For this review, take the finished solid that the model builds, in its own axes (mm). Coordinates: 2 decimals unless noted, no trailing zeros. Loops run counter-clockwise (first coordinate to the right, second up) from the corner with the lowest first, then second, coordinate; pieces in that order, holes last. Notation, with made-up numbers: (67, 9.5) -> (83, 9.5) arc R12 ccw to (83, 26.5) -> close; hole circle Ø8 at (-2, 28.25). An arc over 180 degrees is marked (long way). Use a Markdown table: item, result.
from build123d import *

# Parameters (mm, degrees)
SKETCH1_2_R                 = 1.6383
BOSS_EXTRUDE2_DEPTH         = 1.575
SKETCH2_W                   = 14.080651801
SKETCH2_H                   = 7.11628052
SKETCH2_W_2                 = 15.007196354
SKETCH2_H_2                 = 9.421332762
CUT_EXTRUDE1_DEPTH          = 65.400942629
ADDITIONAL_PCB_MATERIAL_W   = 2.649520344
ADDITIONAL_PCB_MATERIAL_H   = 65.213315835
ADDITIONAL_PCB_MATERIAL_W_2 = 1.5
ADDITIONAL_PCB_MATERIAL_H_2 = 65.299191064
BOSS_EXTRUDE3_DEPTH         = 1.575
SKETCH3_W                   = 46.818
SKETCH3_H                   = 1
BOSS_EXTRUDE4_DEPTH         = 1.575
SKETCH4_W                   = 2
SKETCH4_H                   = 2.5
CUT_EXTRUDE2_DEPTH          = 65.400942629
SKETCH5_W                   = 2.5
SKETCH5_H                   = 18.09999695
SKETCH5_H_2                 = 19.499999394
BOSS_EXTRUDE5_DEPTH         = 1.575
SKETCH7_W                   = 9.5
SKETCH7_H                   = 1.20600305
CUT_EXTRUDE3_DEPTH          = 65.400942629
SKETCH26_W                  = 2.575
SKETCH26_H                  = 5
CUT_EXTRUDE4_DEPTH          = 10


with BuildPart() as part:
    # Sketch1_2 → Boss-Extrude2 (new body)
    with BuildSketch(Plane(origin=(0, 0, 0), x_dir=(1, 0, 0), z_dir=(0, 1, 0))):
        with BuildLine():
            Line((-38.39500299, 29.999999735), (-42.73000299, 29.999999735))
            Line((-42.73000299, 29.999999735), (-43.011025994, 30.003097626))
            ThreePointArc((-43.011025994, 30.003097626), (-43.710996344, 30.299838092), (-44.000003042, 31.003036872))
            Line((-44.000003042, 31.003036872), (-44.000003042, 31.269999735))
            Line((-44.000003042, 31.269999735), (-44.000005679, 44.999999735))
            ThreePointArc((-44.000005679, 44.999999735), (-43.414218633, 46.414215608), (-42.000002924, 47.000003051))
            Line((-42.000002924, 47.000003051), (-30.435003, 47.000003051))
            Line((-30.435003, 47.000003051), (-30.435003, 22.255357341))
            Line((-30.435003, 22.255357341), (-11.409003, 22.255357341))
            Line((-11.409003, 22.255357341), (-11.409003, -9.899999999))
            Line((-11.409003, -9.899999999), (-23.409003, -9.899999999))
            Line((-23.409003, -9.899999999), (-23.409003, -31.499996949))
            Line((-23.409003, -31.499996949), (23.408997, -31.499996949))
            Line((23.408997, -31.499996949), (23.408997, -8.499997555))
            Line((23.408997, -8.499997555), (11.97084713, -8.499997555))
            Line((11.97084713, -8.499997555), (11.97084713, 22.255357341))
            Line((11.97084713, 22.255357341), (30.434997, 22.255357341))
            Line((30.434997, 22.255357341), (30.434997, 47.000003051))
            Line((30.434997, 47.000003051), (42.000008541, 47.000003051))
            ThreePointArc((42.000008541, 47.000003051), (43.414213215, 46.414220704), (43.999996956, 45.000016607))
            Line((43.999996956, 45.000016607), (43.999996956, 32.000003378))
            Line((43.999996956, 32.000003378), (43.999996956, 31.015615364))
            ThreePointArc((43.999996956, 31.015615364), (43.706534093, 30.307939396), (42.998386406, 30.015616661))
            Line((42.998386406, 30.015616661), (33.825607551, 30.030389905))
            ThreePointArc((33.825607551, 30.030389905), (33.117459864, 29.738067169), (32.823997, 29.030391202))
            Line((32.823997, 29.030391202), (32.823997, -30.453996949))
            ThreePointArc((32.823997, -30.453996949), (33.116890219, -31.16110373), (33.823997, -31.453996949))
            Line((33.823997, -31.453996949), (36.099999555, -31.453996949))
            Line((36.099999555, -31.453996949), (42.849728118, -31.453996949))
            ThreePointArc((42.849728118, -31.453996949), (43.556834899, -31.746890168), (43.849728118, -32.453996949))
            Line((43.849728118, -32.453996949), (43.849728118, -36.999996949))
            Line((43.849728118, -36.999996949), (43.849728118, -46.999996949))
            Line((43.849728118, -46.999996949), (-42.000000178, -46.999996949))
            ThreePointArc((-42.000000178, -46.999996949), (-43.414212804, -46.414211581), (-44.000000499, -44.999999921))
            Line((-44.000000499, -44.999999921), (-44.000000178, -38.976999921))
            Line((-44.000000178, -38.976999921), (-44.000000178, -32.453999802))
            ThreePointArc((-44.000000178, -32.453999802), (-43.70710696, -31.746893021), (-43.000000178, -31.453999802))
            Line((-43.000000178, -31.453999802), (-36.100000549, -31.453999802))
            Line((-36.100000549, -31.453999802), (-33.824003042, -31.453999802))
            ThreePointArc((-33.824003042, -31.453999802), (-33.116896261, -31.161106583), (-32.824003042, -30.453999802))
            Line((-32.824003042, -30.453999802), (-32.824003042, 29.011483943))
            ThreePointArc((-32.824003042, 29.011483943), (-33.117785331, 29.719478678), (-33.826516131, 30.011480785))
            Line((-33.826516131, 30.011480785), (-38.39500299, 29.999999735))
        make_face()
        with Locations(Location((40, 43.5, 0), (0, 0, 270))):
            Circle(SKETCH1_2_R, mode=Mode.SUBTRACT)
        with Locations(Location((-40, 43.5, 0), (0, 0, 270))):
            Circle(SKETCH1_2_R, mode=Mode.SUBTRACT)
        with Locations(Location((-37.6, -42.2, 0), (0, 0, 270))):
            Circle(SKETCH1_2_R, mode=Mode.SUBTRACT)
        with Locations(Location((36.1, -42.2, 0), (0, 0, 270))):
            Circle(SKETCH1_2_R, mode=Mode.SUBTRACT)
    extrude(amount=BOSS_EXTRUDE2_DEPTH)

    # Sketch2 → Cut-Extrude1 (cut, through all)
    with BuildSketch(Plane(origin=(0, 1.575, 0), x_dir=(1, 0, 0), z_dir=(0, 1, 0))):
        with Locations((39.863054019, -29.135856689)):
            Rectangle(SKETCH2_W, SKETCH2_H)
        with Locations((-40.336598676, -27.983330568)):
            Rectangle(SKETCH2_W_2, SKETCH2_H_2)
    extrude(amount=-CUT_EXTRUDE1_DEPTH, mode=Mode.SUBTRACT)

    # Additional PCB material → Boss-Extrude3 (add)
    with BuildSketch(Plane(origin=(0, 1.575, 0), x_dir=(1, 0, 0), z_dir=(0, 1, 0))):
        with Locations((32.999236828, -1.128517583)):
            Rectangle(ADDITIONAL_PCB_MATERIAL_W, ADDITIONAL_PCB_MATERIAL_H)
        with Locations((-33.574003042, -1.085579968)):
            Rectangle(ADDITIONAL_PCB_MATERIAL_W_2, ADDITIONAL_PCB_MATERIAL_H_2)
    extrude(amount=-BOSS_EXTRUDE3_DEPTH)

    # Sketch3 → Boss-Extrude4 (add)
    with BuildSketch(Plane(origin=(0, 1.575, 0), x_dir=(1, 0, 0), z_dir=(0, 1, 0))):
        with Locations((-3e-06, -30.999996949)):
            Rectangle(SKETCH3_W, SKETCH3_H)
    extrude(amount=-BOSS_EXTRUDE4_DEPTH)

    # Sketch4 → Cut-Extrude2 (cut, through all)
    with BuildSketch(Plane(origin=(0, 1.575, 0), x_dir=(1, 0, 0), z_dir=(0, 1, 0))):
        with Locations((24.408997, -29.249996949)):
            Rectangle(SKETCH4_W, SKETCH4_H)
        with Locations((-24.409003, -29.249996949)):
            Rectangle(SKETCH4_W, SKETCH4_H)
    extrude(amount=-CUT_EXTRUDE2_DEPTH, mode=Mode.SUBTRACT)

    # Sketch5 → Boss-Extrude5 (add)
    with BuildSketch(Plane(origin=(0, 1.575, 0), x_dir=(1, 0, 0), z_dir=(0, 1, 0))):
        with Locations((-22.159003, -18.949998474)):
            Rectangle(SKETCH5_W, SKETCH5_H)
        with Locations((22.158997, -18.249997252)):
            Rectangle(SKETCH5_W, SKETCH5_H_2)
    extrude(amount=-BOSS_EXTRUDE5_DEPTH)

    # Sketch7 → Cut-Extrude3 (cut, through all)
    with BuildSketch(Plane(origin=(0, 1.575, 0), x_dir=(1, 0, 0), z_dir=(0, 1, 0))):
        with Locations((-16.159003, -9.296998474)):
            Rectangle(SKETCH7_W, SKETCH7_H)
    extrude(amount=-CUT_EXTRUDE3_DEPTH, mode=Mode.SUBTRACT)

    # Sketch26 → Cut-Extrude4 (cut)
    with BuildSketch(Plane(origin=(0, 1.575, 0), x_dir=(1, 0, 0), z_dir=(0, 1, 0))):
        Polygon((-36.984003042, 35.010230552), (-34.324003042, 35.010230552), (-34.324003042, 29.927765717), (-36.984003042, 29.927765717), (-36.984003042, 30.010230552), align=None)
        with Locations((35.612496956, 32.515616661)):
            Rectangle(SKETCH26_W, SKETCH26_H)
    extrude(amount=-CUT_EXTRUDE4_DEPTH, mode=Mode.SUBTRACT)


solid = part.part
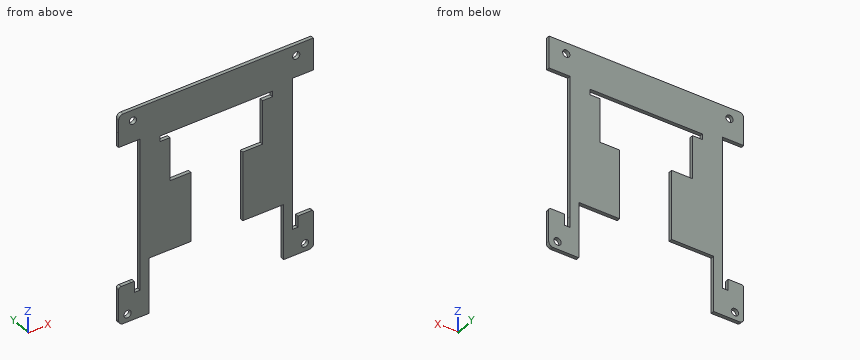
(1) Take a section at A-A on x = -12.5. Write out the cut boundary in (y, z) (3 decimals), plus the area to 3 significant figures.
Found:
| item | result |
|---|---|
| outline | (0, -22.255) -> (1.575, -22.255) -> (1.575, 8.694) -> (0, 8.694) -> close; (0, 30.5) -> (1.575, 30.5) -> (1.575, 47) -> (0, 47) -> close |
| area | 74.7 mm^2 |
(2) Take a section at D-D on x = 40. Write out the cut boundary in (y, z) (3 decimals).
Found:
| item | result |
|---|---|
| outline | (0, -47) -> (1.575, -47) -> (1.575, -45.138) -> (0, -45.138) -> close; (0, -41.862) -> (1.575, -41.862) -> (1.575, -30.02) -> (0, -30.02) -> close; (0, 32.694) -> (1.575, 32.694) -> (1.575, 47) -> (0, 47) -> close |
(3) For line 1 along X through (y, z) = (1, 42.2); line 2 along X through (y, z) = (0.55, -43.5) (3 decimals); line 3 along X through (y, z) = (0.15, 3), list the stretches that pass through material, from the lowest coordinate up.
Found:
| item | result |
|---|---|
| line 1 | x = -44 to -39.24, -35.96 to 34.46, 37.74 to 43.85 |
| line 2 | x = -44 to -41.638, -38.362 to -30.435, 30.435 to 38.362, 41.638 to 44 |
| line 3 | x = -34.32 to -11.41, 11.97 to 34.32 |
(4) For pin 1 Ø0.5 at (y, z) = (1, 18) entering from -X; pin 2 Ø0.8 at (y, z) = (1, -7) entering from +X; pin 3 Ø0.5 at (x, y) = (-5.5, 1) entering from -Z, all flat-tipped, find the tip position at first contact; note any pin that passes through.
Found:
| item | result |
|---|---|
| pin 1 | stops at x = -34.32 |
| pin 2 | stops at x = 34.32 |
| pin 3 | stops at z = 30.5 |
(5) Take a section at C-C on y = 1.3. State how many separate pieces and enclosed holes the cut face has, plus the area to 3 significant figures.
Found:
| item | result |
|---|---|
| separate pieces | 1 |
| enclosed holes | 4 |
| area | 3,830 mm^2 |
(6) Take a section at B-B on z = -26. Write out the cut boundary in (x, y) (3 decimals).
Found:
| item | result |
|---|---|
| outline | (-34.324, 0) -> (-30.435, 0) -> (-30.435, 1.575) -> (-34.324, 1.575) -> close; (30.435, 0) -> (34.324, 0) -> (34.324, 1.575) -> (30.435, 1.575) -> close |
